Solid Edge part; units mm, degrees
sketch "Sketch1" plane through (0, 16.012, 0) normal (0, -1, 0) x (1, 0, 0)
  circle A0 centre (-40.9825, 4.7816) radius 25
extrude "Protrusion1" add sketch "Sketch1" against normal blind 2
sketch "Sketch2" plane through (-40.9825, 18.012, 4.7816) normal (0, 1, 0) x (-1, 0, 0)
  circle A0 centre (0, 0) radius 19.5
extrude "ExtrudedProtrusion_2" add sketch "Sketch2" along normal blind 6
sketch "Sketch3" plane through (-40.9825, 24.012, 4.7816) normal (0, 1, 0) x (-1, 0, 0)
  circle A0 centre (0, 0) radius 25
extrude "ExtrudedProtrusion_3" add sketch "Sketch3" along normal blind 2
sketch "Sketch4" plane through (0, 16.012, 0) normal (0, -1, 0) x (1, 0, 0)
  line L0 (-39.6249, 14.0146) -> (-47.4069, 22.165)
  arc A0 (-47.4069, 22.165) -> (-54.3209, 17.6479) centre (-50.4446, 19.2646) ccw
  line L1 (-54.3209, 17.6479) -> (-49.9832, 7.2473)
  arc A1 (-49.9832, 7.2473) -> (-50.2155, 6.1391) centre (-50.9061, 6.8624) cw
  line L2 (-50.2155, 6.1391) -> (-58.3659, -1.6428)
  arc A2 (-58.3659, -1.6428) -> (-53.8487, -8.5569) centre (-55.4655, -4.6805) ccw
  line L3 (-53.8487, -8.5569) -> (-43.4482, -4.2191)
  arc A3 (-43.4482, -4.2191) -> (-42.34, -4.4515) centre (-43.0633, -5.142) cw
  line L4 (-42.34, -4.4515) -> (-34.5581, -12.6018)
  arc A4 (-34.5581, -12.6018) -> (-27.644, -8.0847) centre (-31.5204, -9.7014) ccw
  line L5 (-27.644, -8.0847) -> (-31.9818, 2.3158)
  arc A5 (-31.9818, 2.3158) -> (-31.7494, 3.424) centre (-31.0588, 2.7008) cw
  line L6 (-31.7494, 3.424) -> (-23.5991, 11.206)
  arc A6 (-23.5991, 11.206) -> (-28.1162, 18.1201) centre (-26.4995, 14.2437) ccw
  line L7 (-28.1162, 18.1201) -> (-38.5167, 13.7823)
  arc A7 (-38.5167, 13.7823) -> (-39.6249, 14.0146) centre (-38.9017, 14.7052) cw
  line L8 (-38.6527, 15.8925) -> (-45.9604, 23.5461)
  arc A8 (-45.9604, 23.5461) -> (-56.1668, 16.878) centre (-50.4446, 19.2646) ccw
  line L9 (-56.1668, 16.878) -> (-52.0934, 7.1114)
  line L10 (-52.0934, 7.1114) -> (-59.747, -0.1963)
  arc A9 (-59.747, -0.1963) -> (-53.0789, -10.4028) centre (-55.4655, -4.6805) ccw
  line L11 (-53.0789, -10.4028) -> (-43.3122, -6.3294)
  line L12 (-43.3122, -6.3294) -> (-36.0046, -13.983)
  arc A10 (-36.0046, -13.983) -> (-25.7981, -7.3148) centre (-31.5204, -9.7014) ccw
  line L13 (-25.7981, -7.3148) -> (-29.8715, 2.4518)
  line L14 (-29.8715, 2.4518) -> (-22.2179, 9.7595)
  arc A11 (-22.2179, 9.7595) -> (-28.8861, 19.966) centre (-26.4995, 14.2437) ccw
  line L15 (-28.8861, 19.966) -> (-38.6527, 15.8925)
extrude "ExtrudedProtrusion_4" add sketch "Sketch4" along normal blind 2
fillet "Round_1" radius 1.5 16 edges at (-60.6559, 16.012, -8.0716) (-48.1956, 16.012, -8.3661) (-55.9202, 16.012, 3.4575) (-39.6584, 16.012, -10.1562) (-28.1293, 16.012, -14.8918) (-27.8348, 16.012, -2.4315) (-43.3122, 15.012, -6.3294) (-29.8715, 15.012, 2.4518) (-26.0447, 16.012, 6.1056) (-21.309, 16.012, 17.6348) (-33.7694, 16.012, 17.9293) (-38.6527, 15.012, 15.8925) (-42.3065, 16.012, 19.7193) (-53.8356, 16.012, 24.455) (-54.1301, 16.012, 11.9947) (-52.0934, 15.012, 7.1114)
sketch "Sketch5" plane through (0, 16.012, 0) normal (0, -1, 0) x (1, 0, 0)
  circle A0 centre (-40.9825, 4.7816) radius 2.75
extrude "Cutout1" cut sketch "Sketch5" against normal up to vertex (10 mm away)
sketch "Sketch6" plane through (0, 16.012, 0) normal (0, -1, 0) x (1, 0, 0)
  circle A0 centre (-30.2039, 11.8235) radius 0.625
  circle A1 centre (-48.0244, 15.5601) radius 0.625
  circle A2 centre (-54.2725, -3.9011) radius 0.625
  circle A3 centre (-33.9406, -5.9969) radius 0.625
extrude "Cutout2" cut sketch "Sketch6" against normal up to vertex (10 mm away)
sketch "Sketch7" plane through (-40.9825, 14.012, 4.7816) normal (0, -1, 0) x (0.9229, 0, 0.3849)
  arc A0 (-5.7404, -7.358) -> (-4.8071, -7.999) centre (-5.7404, -8.358) cw
  line L0 (-4.8071, -7.999) -> (-0.7621, -18.5169)
  arc A1 (-0.7621, -18.5169) -> (7.358, -17.0093) centre (3.158, -17.0093) ccw
  line L1 (7.358, -17.0093) -> (7.358, -5.7404)
  arc A2 (7.358, -5.7404) -> (7.999, -4.8071) centre (8.358, -5.7404) cw
  line L2 (7.999, -4.8071) -> (18.5169, -0.7621)
  arc A3 (18.5169, -0.7621) -> (17.0093, 7.358) centre (17.0093, 3.158) ccw
  line L3 (17.0093, 7.358) -> (5.7404, 7.358)
  arc A4 (5.7404, 7.358) -> (4.8071, 7.999) centre (5.7404, 8.358) cw
  line L4 (4.8071, 7.999) -> (0.7621, 18.5169)
  arc A5 (0.7621, 18.5169) -> (-7.358, 17.0093) centre (-3.158, 17.0093) ccw
  line L5 (-7.358, 17.0093) -> (-7.358, 5.7404)
  arc A6 (-7.358, 5.7404) -> (-7.999, 4.8071) centre (-8.358, 5.7404) cw
  line L6 (-7.999, 4.8071) -> (-18.5169, 0.7621)
  arc A7 (-18.5169, 0.7621) -> (-17.0093, -7.358) centre (-17.0093, -3.158) ccw
  line L7 (-17.0093, -7.358) -> (-5.7404, -7.358)
  arc A8 (-5.7404, -5.858) -> (-3.407, -7.4606) centre (-5.7404, -8.358) cw
  line L8 (-3.407, -7.4606) -> (0.6379, -17.9785)
  arc A9 (0.6379, -17.9785) -> (5.858, -17.0093) centre (3.158, -17.0093) ccw
  line L9 (5.858, -17.0093) -> (5.858, -5.7404)
  arc A10 (5.858, -5.7404) -> (7.4606, -3.407) centre (8.358, -5.7404) cw
  line L10 (7.4606, -3.407) -> (17.9785, 0.6379)
  arc A11 (17.9785, 0.6379) -> (17.0093, 5.858) centre (17.0093, 3.158) ccw
  line L11 (17.0093, 5.858) -> (5.7404, 5.858)
  arc A12 (5.7404, 5.858) -> (3.407, 7.4606) centre (5.7404, 8.358) cw
  line L12 (3.407, 7.4606) -> (-0.6379, 17.9785)
  arc A13 (-0.6379, 17.9785) -> (-5.858, 17.0093) centre (-3.158, 17.0093) ccw
  line L13 (-5.858, 17.0093) -> (-5.858, 5.7404)
  arc A14 (-5.858, 5.7404) -> (-7.4606, 3.407) centre (-8.358, 5.7404) cw
  line L14 (-7.4606, 3.407) -> (-17.9785, -0.6379)
  arc A15 (-17.9785, -0.6379) -> (-17.0093, -5.858) centre (-17.0093, -3.158) ccw
  line L15 (-17.0093, -5.858) -> (-5.7404, -5.858)
extrude "Protrusion2" add sketch "Sketch7" against normal up to vertex (2 mm away)
sketch "Sketch8" plane through (-40.9825, 14.012, 4.7816) normal (0, -1, 0) x (0.9229, 0, 0.3849)
  circle A0 centre (0, 0) radius 32.9501
extrude "ExtrudedCutout_4" cut sketch "Sketch8" against normal blind 7
sketch "Sketch9" plane through (-40.9825, 21.012, 4.7816) normal (0, -1, 0) x (0, 0, 1)
  line L0 (-1.547, 2.3679) -> (0.9156, 14.1125)
  line L1 (4.8305, 13.2916) -> (0.9156, 14.1125)
  line L2 (2.3679, 1.547) -> (4.8305, 13.2916)
  line L3 (2.3679, 1.547) -> (14.1125, -0.9156)
  line L4 (14.1125, -0.9156) -> (13.2916, -4.8305)
  line L5 (1.547, -2.3679) -> (13.2916, -4.8305)
  line L6 (1.547, -2.3679) -> (-0.9156, -14.1125)
  line L7 (-4.8305, -13.2916) -> (-0.9156, -14.1125)
  line L8 (-2.3679, -1.547) -> (-4.8305, -13.2916)
  line L9 (-2.3679, -1.547) -> (-14.1125, 0.9156)
  line L10 (-13.2916, 4.8305) -> (-14.1125, 0.9156)
  line L11 (-1.547, 2.3679) -> (-13.2916, 4.8305)
  circle A0 centre (0, 0) radius 2.75
extrude "ExtrudedProtrusion_6" add sketch "Sketch9" along normal blind 2
properties material "ABS Plastic, medium impact"
Here's how the part is built. I have some questions about the finished solid (model axes, mm). A direction names the side the tool comes from. Give positions to 0.01 mm unless a question says otherwise; leave off trailing zeros. Order: outer loops, then holes, each group sorted by start corner. A loop starts at its lowest first (then second) coordinate and runs counter-clockwise, first axis right, second up. Notation, with made-up numbers: M -8,-10 L 45,-10 A13 ccw 45,14 Z; hole C 21,-24.75 d9. An arc over 180 degrees is marked long. Answer as a JSON object with one key per item and string values. Group by question number.
1) Suppose I cut it at D-D, the plane x = -26. Write out the boundary of the cut face in (y, z), plus the area to 3 significant figures.
2) Suppose I cut it at C-C, the plane z = -12. Write out the boundary of the cut face in (x, y), plus the area to 3 significant figures.
3) I'm going to push flat-ended pins straight in: pin 1 Ø2 at (x, z) = (-50, 16.5) entering from -Y; pin 2 Ø1.5 at (y, z) = (25, 24) entering from +X; pin 3 Ø1.5 at (x, y) = (-57, 23) entering from -Z; pin 4 Ø1.1 at (x, z) = (-30.2, 11.82) entering from +Y. Where does each tip first touch, or does it pass through?
4) Suppose I cut it at B-B, the plane x = -48. Write out the boundary of the cut face in (y, z).
5) Please list where these lines run through material, in increasing order: L1, parallel to Y at x = -59.5, z = 14; L2, parallel to Y at x = -59.5, z = 5; L3, parallel to Z at x = -39, y = 19.75. Write a range as [from, to].
6) We'd pull the mould along Z, two halves only. Please class faces 4 (the flat face through (-48.32, 20.026, 8.364)), 5 (the flat face through (-44.564, 20.026, -2.555)), 6 (the flat face through (-56, 24.012, -8)), 7 (the flat face through (-27.286, 20.026, 1.881)): pulls with the +Z half, pulls with the -Z half, needs draft (parallel to the pull), parting line crosses it, or undercut.
7) On a 3-axis mill with a long thin cutter (end or side, diameter ignored), from which of +Z, -Z, +X, -X, +Y, -Y can I reach the whole of each face in a straight line? I mean faces 1 (the flat face through (-43.883, 20.026, -8.915)), 2 (the flat face through (-40.65, 20.03, -3.38)), 3 (the flat face through (-38.14, 20.03, 18.49)). Say none if no direction works.
Results found:
{
 "1": {"outline": "M 21.01,-7.7 L 24.01,-7.7 L 24.01,-15.23 L 26.01,-15.23 L 26.01,24.79 L 24.01,24.79 L 24.01,17.26 L 21.01,17.26 Z", "area": "155 mm²"},
 "2": {"outline": "M -59.51,24.01 L -50.91,24.01 L -50.91,21.01 L -31.05,21.01 L -31.05,24.01 L -22.45,24.01 L -22.45,26.01 L -59.51,26.01 Z", "area": "134 mm²"},
 "3": {"pin 1": "y = 21.01", "pin 2": "x = -24.13", "pin 3": "z = -7.35", "pin 4": "through"},
 "4": {"outline": "M 19.01,4.21 L 21.01,4.21 L 21.01,-13.41 L 24.01,-13.41 L 24.01,-19.21 L 26.01,-19.21 L 26.01,14.94 L 21.01,14.94 L 21.01,8.3 L 19.01,8.3 Z; M 21.01,16.18 L 26.01,16.18 L 26.01,28.78 L 24.01,28.78 L 24.01,22.98 L 21.01,22.98 Z"},
 "5": {"L1": "[24.01, 26.01]", "L2": "[21.01, 26.01]", "L3": "[2.32, 2.88], [6.69, 18.67]"},
 "6": {"face 4": "pulls with the +Z half", "face 5": "undercut", "face 6": "needs draft", "face 7": "pulls with the -Z half"},
 "7": {"face 1": "-Z, -X, -Y", "face 2": "-Z, -Y", "face 3": "+Z, +X, -Y"}
}
